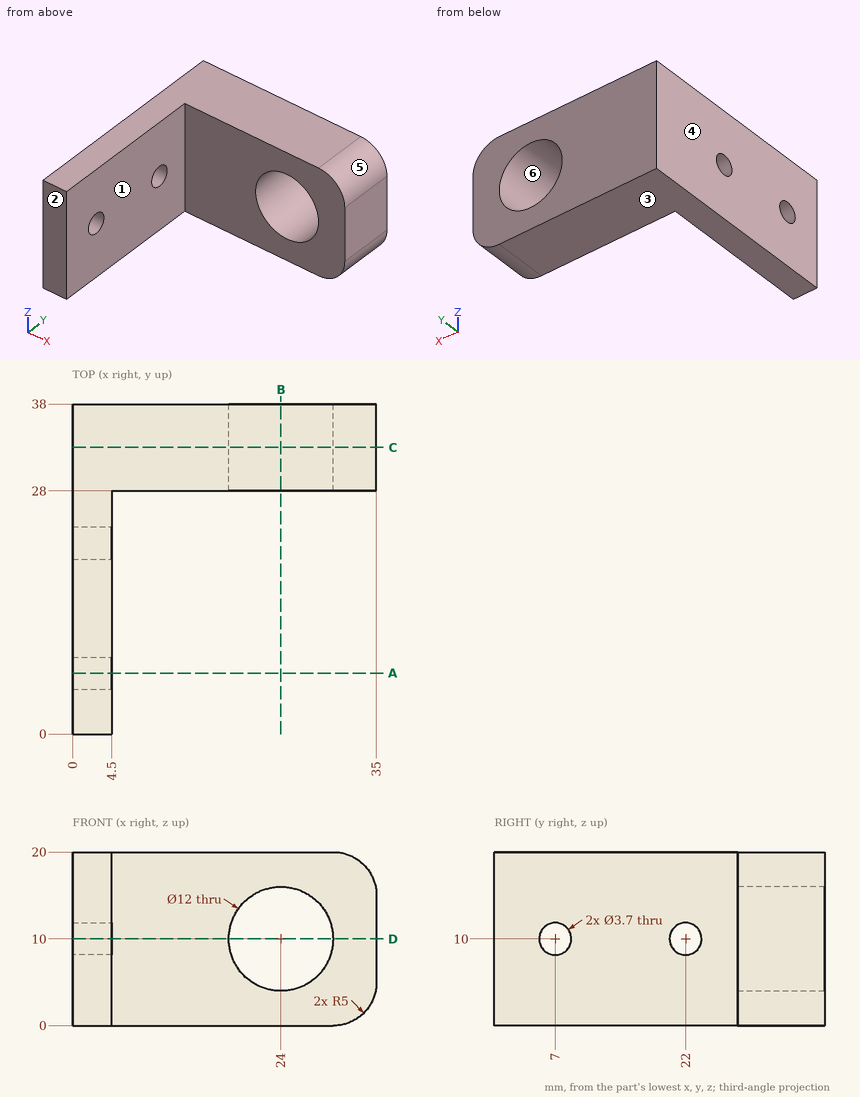
Can you work these out from the drawing? Everything is in mm from the part's minimum corner. A direction names the side the tool comes from. Round coordinates to 2 decimals unless told otherwise and drop trailing zeros. Order: outer loops, then holes, each group sorted by start corner. A loop starts at its lowest first (then second) coordinate and runs counter-clockwise, first axis right, second up. Notation, with made-up numbers: (14.5, -25.75) - (62.5, -25.75) arc R14 ccw to (62.5, -6.75) - close; hole circle Ø4 at (38.5, -39). An arc over 180 degrees is marked (long way). Answer in a Markdown table with one row per item.
(1) Suppose I cut it at B-B, the plane x = 24. Please give me the cut outline in (y, z).
From the geometry:
| item | result |
|---|---|
| outline | (28, 0) - (38, 0) - (38, 4) - (28, 4) - close; (28, 16) - (38, 16) - (38, 20) - (28, 20) - close |
(2) For P1, Ø5, axis at y = 19, z = 15, coming from the +X side; P2, Ø3.5, axis at y = 22, z = 10, coming from the +X side; P3, Ø8, axis at y = 13, z = 13, coming from the -X side; P4, Ø5, axis at x = 20, z = 6.5, coming from the -Y side, each with a flat end and sliding along its axis, tell me the tip position at first contact or that it passes through.
From the geometry:
| item | result |
|---|---|
| P1 | stops at x = 4.5 |
| P2 | passes through |
| P3 | stops at x = 0 |
| P4 | stops at y = 28 |
(3) If we mould it in two halves opening along X, with no side actions, what happens to the marked faces 3, 4, 5 and 6? For each: released by +X, released by -X, zero draft, split by the parting line, or undercut.
From the geometry:
| item | result |
|---|---|
| face 3 | zero draft |
| face 4 | released by -X |
| face 5 | released by +X |
| face 6 | undercut |
(4) Suppose I cut it at C-C, the plane y = 33. Please give me the cut outline in (x, z).
From the geometry:
| item | result |
|---|---|
| outline | (0, 0) - (30, 0) arc R5 ccw to (35, 5) - (35, 15) arc R5 ccw to (30, 20) - (0, 20) - close; hole circle Ø12 at (24, 10) |
(5) Suppose I cut it at A-A, the plane y = 7. Please give me the cut outline in (x, z), plus the area to 4 significant figures.
From the geometry:
| item | result |
|---|---|
| outline | (0, 0) - (4.5, 0) - (4.5, 8.15) - (0, 8.15) - close; (0, 11.85) - (4.5, 11.85) - (4.5, 20) - (0, 20) - close |
| area | 73.35 mm2 |
(6) Which directions (+Z, -Z, +X, -X, +Y, -Y) give clear straight access to the entire face, cutting with the end or side of a thin tool? Please do the marked faces 1 and 2.
From the geometry:
| item | result |
|---|---|
| face 1 | +Z, -Z, +X, -Y |
| face 2 | +Z, -Z, +X, -X, -Y |
(7) Suppose I cut it at D-D, the plane z = 10. Please give me the cut outline in (x, y), plus the area to 3 significant figures.
From the geometry:
| item | result |
|---|---|
| outline | (0, 0) - (4.5, 0) - (4.5, 5.15) - (0, 5.15) - close; (0, 8.85) - (4.5, 8.85) - (4.5, 20.15) - (0, 20.15) - close; (0, 23.85) - (4.5, 23.85) - (4.5, 28) - (18, 28) - (18, 38) - (0, 38) - close; (30, 28) - (35, 28) - (35, 38) - (30, 38) - close |
| area | 323 mm2 |
(8) Please list where these lines run through material, in increasing order: L1, parallel to Y at x = 2.45, z = 10; L2, parallel to X at y = 30.5, z = 10; L3, parallel to Y at x = 28, z = 15.75. Write a range as from..to.
From the geometry:
| item | result |
|---|---|
| L1 | y = 0..5.15, 8.85..20.15, 23.85..38 |
| L2 | x = 0..18, 30..35 |
| L3 | y = 28..38 |
